```python
from build123d import *

# Parameters (mm, degrees)
SKETCH1_W           = 71.12
SKETCH1_H           = 63.5
INNER_LID_DEPTH     = 3.81
SKETCH1_5_W         = 78.74
SKETCH1_5_H         = 71.12
SKETCH1_5_W_2       = 71.12
SKETCH1_5_H_2       = 63.5
OUTER_LID_DEPTH     = 6.35
SKETCH2_W           = 2.54
SKETCH2_H           = 6.35
HOLE_SLIDES_DEPTH   = 11.43
SKETCH3_R           = 4.445
HOLE_LID_1_DEPTH    = 3.81
BOSS_EXTRUDE5_START = -3.81
SKETCH4_R           = 4.445
BOSS_EXTRUDE5_DEPTH = 3.81


with BuildPart() as part:
    # Sketch1 → inner-lid (new body)
    with BuildSketch(Plane(origin=(0, 0, 0), x_dir=(1, 0, 0), z_dir=(0, 1, 0))):
        Rectangle(SKETCH1_W, SKETCH1_H)
    extrude(amount=INNER_LID_DEPTH)

    # Sketch1<5> → outer-lid (add)
    with BuildSketch(Plane(origin=(0, 0, 0), x_dir=(1, 0, 0), z_dir=(0, 1, 0))):
        Rectangle(SKETCH1_5_W, SKETCH1_5_H)
        Rectangle(SKETCH1_5_W_2, SKETCH1_5_H_2, mode=Mode.SUBTRACT)
    extrude(amount=OUTER_LID_DEPTH)

    # Sketch2 → hole-slides (add)
    with BuildSketch(Plane(origin=(0, 6.35, 0), x_dir=(1, 0, 0), z_dir=(0, 1, 0))):
        with Locations((36.83, 0)):
            Rectangle(SKETCH2_W, SKETCH2_H)
        with Locations((-36.83, 0)):
            Rectangle(SKETCH2_W, SKETCH2_H)
    extrude(amount=HOLE_SLIDES_DEPTH)

    # Sketch3 → hole-lid-1 (add)
    with BuildSketch(Plane(origin=(-35.56, 0, 0), x_dir=(0, 0, -1), z_dir=(1, 0, 0))):
        with Locations((0, 17.78)):
            Circle(SKETCH3_R)
    extrude(amount=-HOLE_LID_1_DEPTH)

    # Sketch4 → Boss-Extrude5 (add)
    with BuildSketch(Plane.ZY.offset(-35.56).offset(BOSS_EXTRUDE5_START)):
        with Locations(Location((0, 17.78, 0), (0, 0, 180))):
            Circle(SKETCH4_R)
    extrude(amount=BOSS_EXTRUDE5_DEPTH)


solid = part.part
```
Build history of the part. All positions in model axes, mm. A direction names the side the tool comes from. Round coordinates to 2 decimals unless told otherwise and drop trailing zeros. Order: outer loops, then holes, each group sorted by start corner. A loop starts at its lowest first (then second) coordinate and runs counter-clockwise, first axis right, second up. Notation, with made-up numbers: (6, 30) -> (44, 30) arc R35 cw to (44, 65) -> close; hole circle Ø11 at (51.5, 67). An arc over 180 degrees is marked (long way). Answer in a Markdown table with one row per item.
1) Band-saw the part on C-C on z = 0. Give the cut face in (x, y) (3 decimals), and give its area (3 significant figures).
Values:
| item | result |
|---|---|
| outline | (-39.37, 0) -> (39.37, 0) -> (39.37, 6.35) -> (38.1, 6.35) -> (38.1, 13.335) -> (39.37, 13.335) -> (39.37, 22.225) -> (35.56, 22.225) -> (35.56, 3.81) -> (-35.56, 3.81) -> (-35.56, 22.225) -> (-39.37, 22.225) -> (-39.37, 13.335) -> (-38.1, 13.335) -> (-38.1, 6.35) -> (-39.37, 6.35) -> close |
| area | 423 mm2 |
2) Wall check: L1, parallel to Z at x = 8, y = 4.5; L2, parallel to X at y = 5.75, z = 24; L3, parallel to Y at x = -20, z = -12. Give the ranges that are in metal, low to high.
Values:
| item | result |
|---|---|
| L1 | -35.56 to -31.75, 31.75 to 35.56 |
| L2 | -39.37 to -35.56, 35.56 to 39.37 |
| L3 | 0 to 3.81 |
3) Band-saw the part on B-B on x = 20. Give the cut face in (y, z).
Values:
| item | result |
|---|---|
| outline | (0, -35.56) -> (6.35, -35.56) -> (6.35, -31.75) -> (3.81, -31.75) -> (3.81, 31.75) -> (6.35, 31.75) -> (6.35, 35.56) -> (0, 35.56) -> close |
4) Band-saw the part on A-A on y = 17.78. Give the cut face in (x, z) (3 decimals).
Values:
| item | result |
|---|---|
| outline | (-39.37, -4.445) -> (-35.56, -4.445) -> (-35.56, 4.445) -> (-39.37, 4.445) -> close; (35.56, -4.445) -> (39.37, -4.445) -> (39.37, 4.445) -> (35.56, 4.445) -> close |
5) Mould opens along Y. For faces 1 (the flat face through (0, 3.81, 0)), 2 (the flat face through (-39.37, 18, 0)), 3 (the flat face through (-38.1, 10, 0)) say: released by +Y, released by -Y, zero draft, split by the parting line, or undercut.
Values:
| item | result |
|---|---|
| face 1 | released by +Y |
| face 2 | zero draft |
| face 3 | undercut |
6) Band-saw the part on D-D on z = 22.5. Give the cut face in (x, y).
Values:
| item | result |
|---|---|
| outline | (-39.37, 0) -> (39.37, 0) -> (39.37, 6.35) -> (35.56, 6.35) -> (35.56, 3.81) -> (-35.56, 3.81) -> (-35.56, 6.35) -> (-39.37, 6.35) -> close |
7) Which spindle directions (+Z, -Z, +X, -X, +Y, -Y) get a long thin tool onto all of the face, cutting with end or side? Do faces 4 (the flat face through (35.56, 9, 0)), 5 (the flat face through (-37, 10, 3.175)), 6 (the flat face through (-37, 10, -3.175)). Say none if no direction does.
Values:
| item | result |
|---|---|
| face 4 | +Y |
| face 5 | +Z, +X, -X |
| face 6 | -Z, +X, -X |
8) Pin check, flat tips, straight feed: P1, Ø0.8, axis at x = 37, y = 10, coming from the -Z side (3 decimals); P2, Ø1.3, axis at x = -37.5, y = 9.5, coming from the +Z side (3 decimals); P3, Ø5.5, axis at y = 13, z = -5.5, coming from the +X side. Stop position of each tip, or through.
Values:
| item | result |
|---|---|
| P1 | z = -3.175 |
| P2 | z = 3.175 |
| P3 | x = 38.1 |
